```python
from build123d import *

# Parameters (mm, degrees)
F0_W     = 50.8
F0_H     = 50.8
F2_DEPTH = 50.8
F1_R     = 12.7
F3_DEPTH = 50.8
F4_R     = 12.7
F5_DEPTH = 12.7
F6_W     = 25.4
F6_H     = 25.4
F7_DEPTH = 25.4


with BuildPart() as f2:
    # F0 (on Front) → F2 (new body)
    with BuildSketch(Plane.XZ):
        with Locations((-25.4, 25.4)):
            Rectangle(F0_W, F0_H)
    extrude(amount=F2_DEPTH)

    # F1 (on Front) → F3 (cut)
    with BuildSketch(Plane.XZ):
        with Locations((-24.174957, 25.38876)):
            Circle(F1_R)
    extrude(amount=F3_DEPTH, mode=Mode.SUBTRACT)

    # F4 (on face) → F5 (join)
    with BuildSketch(Plane(origin=(-50.8, 0, 0), x_dir=(0, -1, 0), z_dir=(-1, 0, 0))):
        with Locations((25.793362, 25.38876)):
            Circle(F4_R)
    extrude(amount=F5_DEPTH)

    # F6 (on Right) → F7 (join)
    with BuildSketch(Plane.YZ):
        with Locations((-28.176018, 27.973717)):
            Rectangle(F6_W, F6_H)
    extrude(amount=F7_DEPTH)


solid = f2.part
```
Verification items for the finished model (mm, model axes). A direction names the side the tool comes from. Coordinates: 2 decimals unless noted, no trailing zeros. Loops run counter-clockwise (first coordinate to the right, second up) from the corner with the lowest first, then second, coordinate; pieces in that order, holes last. Notation, with made-up numbers: (81, -38) - (134, -38) arc R32 ccw to (134, -10) - close; hole circle Ø4 at (80, 35). An arc over 180 degrees is marked (long way). Answer as a JSON object with one key per item and string values.
(1) Cross-section at B-B, the plane x = -34. Record the boundary of the cut face in (y, z).
Response:
{"outline": "(-50.8, 0) - (0, 0) - (0, 17.34) - (-50.8, 17.34) - close; (-50.8, 33.44) - (0, 33.44) - (0, 50.8) - (-50.8, 50.8) - close"}
(2) Cross-section at A-A, the plane z = 27. Record the boundary of the cut face in (x, y).
Response:
{"outline": "(-63.5, -38.39) - (-50.8, -38.39) - (-50.8, -50.8) - (-36.77, -50.8) - (-36.77, 0) - (-50.8, 0) - (-50.8, -13.2) - (-63.5, -13.2) - close; (-11.58, -50.8) - (0, -50.8) - (0, -40.88) - (25.4, -40.88) - (25.4, -15.48) - (0, -15.48) - (0, 0) - (-11.58, 0) - close"}
(3) Cross-section at D-D, the plane z = 10. Record the boundary of the cut face in (x, y), then the cut area to 3 significant figures.
Response:
{"outline": "(-50.8, -50.8) - (0, -50.8) - (0, 0) - (-50.8, 0) - close", "area": "2,580 mm²"}
(4) Cross-section at C-C, the plane y = -32. Record the boundary of the cut face in (x, z), then the cut area to 3 significant figures.
Response:
{"outline": "(-63.5, 14.31) - (-50.8, 14.31) - (-50.8, 0) - (0, 0) - (0, 15.27) - (25.4, 15.27) - (25.4, 40.67) - (0, 40.67) - (0, 50.8) - (-50.8, 50.8) - (-50.8, 36.47) - (-63.5, 36.47) - close; hole circle Ø25.4 at (-24.17, 25.39)", "area": "3,000 mm²"}
(5) Access from +Z, -Z, +X, -X, +Y, -Y to the whole of each face (thin tool, end or side, straight path). Record for faces 1 (the flat face through (13, -40.876, 28)), 2 (the flat face through (13, -28, 15.274)), 3 (the flat face through (-50.8, -14, 19)), 4 (the flat face through (13, -15.476, 28)).
Response:
{"face 1": "+Z, -Z, +X, -Y", "face 2": "-Z, +X, +Y, -Y", "face 3": "-X", "face 4": "+Z, -Z, +X, +Y"}
(6) Go/stop test with flat-tipped pins: pin 1 Ø3 at (x, y) = (9.5, -15.5) entering from -Z; pin 2 Ø7.5 at (x, z) = (17, 30) entering from +Y; pin 3 Ø10 at (x, y) = (7.5, -28.5) entering from +Z; pin 4 Ø4 at (x, y) = (13, -11.5) entering from +Z. Record where each tip stops, or that it passes through.
Response:
{"pin 1": "stops at z = 15.27", "pin 2": "stops at y = -15.48", "pin 3": "stops at z = 40.67", "pin 4": "passes through"}
(7) Mould release check, pull along X, two halves, no side actions. Record for faces 5 (the flat face through (-63.5, -26, 26)), 6 (the flat face through (-37.04, -50.8, 25.76)), 7 (the cylindrical face through (-34.25, -25.04, 17.66)): pulls with the +X half, pulls with the -X half, needs draft (parallel to the pull), parting line crosses it, or undercut.
Response:
{"face 5": "pulls with the -X half", "face 6": "needs draft", "face 7": "undercut"}
(8) Scan lines: line 1 along Z through (x, y) = (-24, -9); line 2 along X through (y, z) = (-46.5, 8); line 3 along X through (y, z) = (-5, 19.5). Record each from-to range of solid material in increasing order.
Response:
{"line 1": "z = 0 to 12.69, 38.09 to 50.8", "line 2": "x = -50.8 to 0", "line 3": "x = -50.8 to -35.43, -12.92 to 0"}
